Model file for the job. Use its own axes, mm. Face numbers are marked on the shaded views. A direction names the side the tool comes from. Round coordinates to 2 decimals unless told otherwise and drop trailing zeros. Loops run counter-clockwise (first coordinate to the right, second up) from the corner with the lowest first, then second, coordinate; pieces in that order, holes last. Notation, with made-up numbers: (46, -12) - (87, -12) arc R22 cw to (87, 6) - close; hole circle Ø10 at (-15, -12.5). An arc over 180 degrees is marked (long way). Use one line per item in the form item = value.
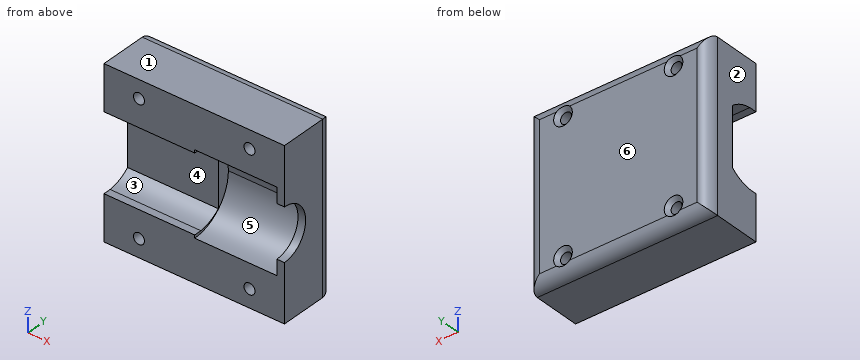
from build123d import *

# Parameters (mm, degrees)
SKETCH1_W           = 47.46
SKETCH1_H           = 44
BOSS_EXTRUDE1_DEPTH = 15.4
SKETCH2_W           = 21.6
SKETCH2_H           = 21.82
CUT_EXTRUDE1_DEPTH  = 10.91
FILLET1_R           = 10.91
SKETCH4_W           = 23.86
SKETCH4_H           = 20.2
CUT_EXTRUDE2_DEPTH  = 7.65
SKETCH8_R           = 1.45
CUT_EXTRUDE3_DEPTH  = 20.18
CHAMFER1_SIZE       = 1
FILLET2_R           = 3
SKETCH9_R           = 6.86
CUT_EXTRUDE4_DEPTH  = 2.18
BOSS_EXTRUDE3_DEPTH = 23.86


# Some blends are built 0.0001 mm under size
with BuildPart() as part:
    # Sketch1 → Boss-Extrude1 (new body)
    with BuildSketch(Plane(origin=(0, 0, 0), x_dir=(1, 0, 0), z_dir=(0, 1, 0))):
        Rectangle(SKETCH1_W, SKETCH1_H)
    extrude(amount=BOSS_EXTRUDE1_DEPTH)

    # Sketch2 → Cut-Extrude1 (cut)
    with BuildSketch(Plane.XZ):
        with Locations((10.93, 0)):
            Rectangle(SKETCH2_W, SKETCH2_H)
    extrude(amount=-CUT_EXTRUDE1_DEPTH, mode=Mode.SUBTRACT)

    # Fillet1
    fillet1_edges = [part.edges().sort_by_distance(p)[0] for p in [
        (10.93, 10.91, -10.91),
        (10.93, 10.91, 10.91),
    ]]
    fillet(fillet1_edges, radius=FILLET1_R - 0.0001)  # a hair under: the kernel refuses the full size

    # Sketch4 → Cut-Extrude2 (cut)
    with BuildSketch(Plane.XZ):
        with Locations((-11.8, 0)):
            Rectangle(SKETCH4_W, SKETCH4_H)
    extrude(amount=-CUT_EXTRUDE2_DEPTH, mode=Mode.SUBTRACT)

    # Sketch8 → Cut-Extrude3 (cut)
    with BuildSketch(Plane.XZ):
        with Locations(Location((14.535, -17.265, 0), (0, 0, 270))):
            Circle(SKETCH8_R)
        with Locations(Location((-14.535, -17.265, 0), (0, 0, 270))):
            Circle(SKETCH8_R)
    cut_extrude3 = extrude(amount=-CUT_EXTRUDE3_DEPTH, mode=Mode.SUBTRACT)

    # Mirror1: Cut-Extrude3 across plane
    add(cut_extrude3.mirror(Plane(origin=(0, 0, 0), x_dir=(1, 0, 0), z_dir=(0, 0, -1))), mode=Mode.SUBTRACT)

    # Chamfer1
    chamfer1_edges = [part.edges().sort_by_distance(p)[0] for p in [
        (14.535, 15.4, -15.815),
        (-14.535, 15.4, -15.815),
        (14.535, 15.4, 15.815),
        (-14.535, 15.4, 15.815),
    ]]
    chamfer(chamfer1_edges, length=CHAMFER1_SIZE)

    # Fillet2
    # the kernel refuses this fillet: 3 mm, written as the material it takes off along each edge
    with BuildSketch(Plane(origin=(23.73, 15.4, 29.5), x_dir=(-1, 0, 0), z_dir=(0, 0, -1)), Plane(origin=(-23.73, 15.4, -29.5), x_dir=(1, 0, 0), z_dir=(0, 0, 1))) as fillet2_piece_1:
        with BuildLine():
            CenterArc((FILLET2_R, -FILLET2_R), FILLET2_R, 90, 90)
            Line((0, -FILLET2_R), (0, 0))
            Line((0, 0), (FILLET2_R, 0))
        make_face()
    extrude(amount=59, mode=Mode.SUBTRACT)
    with BuildSketch(Plane(origin=(31.23, 15.4, -22), x_dir=(0, 0, 1), z_dir=(-1, 0, 0)), Plane(origin=(-31.23, 15.4, 22), x_dir=(0, 0, -1), z_dir=(1, 0, 0))) as fillet2_piece_2:
        with BuildLine():
            CenterArc((FILLET2_R, -FILLET2_R), FILLET2_R, 90, 90)
            Line((0, -FILLET2_R), (0, 0))
            Line((0, 0), (FILLET2_R, 0))
        make_face()
    extrude(amount=62.46, mode=Mode.SUBTRACT)

    # Sketch9 → Cut-Extrude4 (cut)
    with BuildSketch(Plane(origin=(23.73, 0, 0), x_dir=(0, 0, -1), z_dir=(1, 0, 0))):
        Circle(SKETCH9_R)
    extrude(amount=-CUT_EXTRUDE4_DEPTH, mode=Mode.SUBTRACT)

    # Sketch10 → Boss-Extrude3 (add)
    with BuildSketch(Plane.ZY.offset(23.73)):
        with BuildLine():
            Line((-7.65, 7.65), (-10.1, 7.65))
            Line((-10.1, 7.65), (-10.1, 1.997052779))
            ThreePointArc((-10.1, 1.997052779), (-9.316559187, 5.014899131), (-7.65, 7.65))
        make_face()
        with BuildLine():
            Line((10.1, 1.997052779), (10.1, 7.65))
            Line((10.1, 7.65), (7.65, 7.65))
            ThreePointArc((7.65, 7.65), (9.316559187, 5.014899131), (10.1, 1.997052779))
        make_face()
    extrude(amount=-BOSS_EXTRUDE3_DEPTH)


solid = part.part
1. Cut at B-B, the plane y = 13.5. Give the cut face in (x, z) (3 decimals), plus the area to 3 significant figures.
Geometry check:
outline = (-23.521, -21.791) - (23.521, -21.791) - (23.521, 21.791) - (-23.521, 21.791) - close; hole circle Ø2.9 at (-14.535, -17.265); hole circle Ø2.9 at (-14.535, 17.265); hole circle Ø2.9 at (14.535, -17.265); hole circle Ø2.9 at (14.535, 17.265)
area = 2,020 mm^2
2. Cut at A-A, the plane y = 3. Give the cut face in (x, z) (3 decimals), plus the area to 3 significant figures.
Geometry check:
outline = (-23.73, -22) - (23.73, -22) - (23.73, -6.169) - (21.73, -6.169) - (21.73, -10.489) - (0.13, -10.489) - (0.13, -9.949) - (-23.73, -9.949) - close; (-23.73, 9.949) - (0.13, 9.949) - (0.13, 10.489) - (21.73, 10.489) - (21.73, 6.169) - (23.73, 6.169) - (23.73, 22) - (-23.73, 22) - close; hole circle Ø2.9 at (-14.535, -17.265); hole circle Ø2.9 at (-14.535, 17.265); hole circle Ø2.9 at (14.535, -17.265); hole circle Ø2.9 at (14.535, 17.265)
area = 1,110 mm^2
3. Flat gauge pins, fed straight in: pin 1 (12 mm diameter, centred on x = -6.5, z = -0.5, fed in from -Y); pin 2 (4.5 mm diameter, centred on x = -14.535, z = 17.265, fed in from +Y); pin 3 (4.5 mm diameter, centred on x = 14.535, z = 17.265, fed in from -Y). Where does each tip first touch, or does it go through?
Geometry check:
pin_1 = 7.65
pin_2 = 15.2
pin_3 = 0
4. Wall check: probe 1 along Z at (x, y) = (-4.5, 1.5); probe 2 along X at (y, z) = (5.5, -16); probe 3 along Z at (x, y) = (-15.5, 1). Give the ranges that are in metal, low to high.
Geometry check:
probe_1 = -22 to -10.1, 10.1 to 22
probe_2 = -23.73 to -15.24, -13.83 to 13.83, 15.24 to 23.73
probe_3 = -22 to -18.35, -16.18 to -10.1, 10.1 to 16.18, 18.35 to 22
5. Cut at C-C, the plane z = 6. Give the cut face in (x, y).
Geometry check:
outline = (-23.73, 7.65) - (0.13, 7.65) - (0.13, 9.11) - (21.73, 9.11) - (21.73, 3.33) - (23.73, 3.33) - (23.73, 12.4) arc R3 ccw to (20.73, 15.4) - (-20.73, 15.4) arc R3 ccw to (-23.73, 12.4) - close
6. Cut at D-D, the plane z = -16.5. Give the number of separate pieces and of enclosed holes in the cut face, plus the area to 3 significant figures.
Geometry check:
separate_pieces = 3
enclosed_holes = 0
area = 649 mm^2
7. Pull direction Z, two halves, no side cores. Call the marked faces 1, 2 and 3: +Z half, -Z half, draft (parallel to the pull), parting line (faces both ways), or undercut.
Geometry check:
face_1 = +Z half
face_2 = draft
face_3 = undercut
8. Tool access for the marked faces 4, 5 and 6: list every direction of +Z, -Z, +X, -X, +Y, -Y with a clear straight run to the whole face (end or side of a thin tool).
Geometry check:
face_4 = -X, -Y
face_5 = -Y
face_6 = +Z, -Z, +X, -X, +Y
